Autodesk Inventor part; units mm, degrees
ref_plane "YZ Plane" through (0, 0, 0) normal (1, 0, 0) x (0, 1, 0)
ref_plane "XZ Plane" through (0, 0, 0) normal (0, 1, 0) x (-1, 0, 0)
ref_plane "XY Plane" through (0, 0, 0) normal (0, 0, 1) x (1, 0, 0)
sketch "Sketch1" plane through (0, 0, 0) normal (0, 1, 0) x (-1, 0, 0)
  line L0 (-3.6662, 6.35) -> (3.6662, 6.35)
  line L1 (3.6662, 6.35) -> (7.3323, 0)
  line L2 (7.3323, 0) -> (3.6662, -6.35)
  line L3 (3.6662, -6.35) -> (-3.6662, -6.35)
  line L4 (-3.6662, -6.35) -> (-7.3323, 0)
  line L5 (-7.3323, 0) -> (-3.6662, 6.35)
  point P0 (0, 0)
  point P1 (0, 0)
  dimension "d0" = 12.7
extrude "Extrusion1" add sketch "Sketch1" along normal blind 171.45
sketch "Sketch2" plane through (0, 171.45, 0) normal (0, 1, 0) x (1, 0, 0)
  circle A0 centre (0, 0) radius 2.54
  dimension "d3" = 5.08
extrude "Extrusion2" cut sketch "Sketch2" against normal blind 25.4
thread "Thread1"
sketch "Sketch3" plane through (0, 0, 0) normal (0, -1, 0) x (1, 0, 0)
  circle A0 centre (0, 0) radius 2.54
  dimension "d8" = 5.08
extrude "Extrusion3" cut sketch "Sketch3" against normal blind 25.4
thread "Thread2"
properties part number "OUTK_013_Shaft1" material "Aluminum 6061"
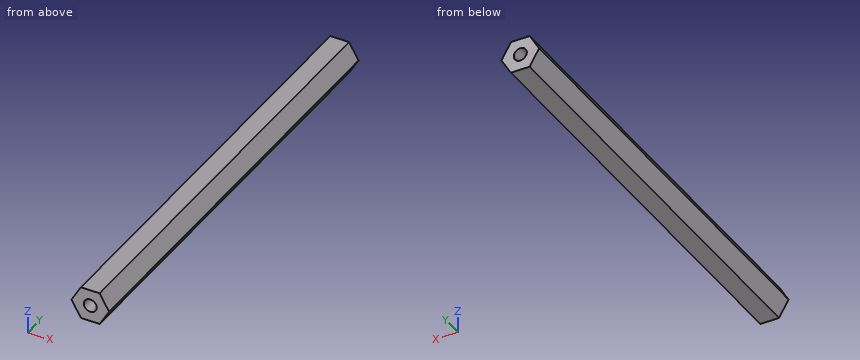
Source: CAD feature listing. Evaluate the final solid. Frame: model axes, mm. Give positions to 0.01 mm unless a question says otherwise; leave off trailing zeros. Loops run counter-clockwise (first coordinate to the right, second up) from the corner with the lowest first, then second, coordinate; pieces in that order, holes last. Notation, with made-up numbers: (42, 50) -> (76, 50) arc R20 ccw to (76, 58) -> close; hole circle Ø1 at (22, -23.75). An arc over 180 degrees is marked (long way). Use a Markdown table: item, result. Add a question column.
1) First-contact query: pin 1 (2.5 mm diameter, centred on x = 1, z = 0, fed in from +Y); pin 2 (4 mm diameter, centred on x = 0, z = 0, fed in from -Y); pin 3 (2 mm diameter, centred on x = 5, y = 51, fed in from +Z). Flat tips, straight axial feed; report the tip coordinate or a pass-through.
2) Section query A-A, the plane y = 150. Return the cut outline in (x, z), then the cut area to 3 significant figures.
3) Section query B-B, the plane y = 58. Return the cut outline in (x, z).
4) Section query C-C, the plane x = 0. Return the cut outline in (y, z).
5) Line query: line 1 along X through (y, z) = (152, 0); line 2 along Z through (x, y) = (0, 17.5); line 3 along Y through (x, z) = (-1.5, -2). Output: solid intervals per line, ascending. Write a range as [from, to].
Numbers:
| question | item | result |
|---|---|---|
| 1 | pin 1 | stops at y = 146.05 |
| 1 | pin 2 | stops at y = 25.4 |
| 1 | pin 3 | stops at z = 5.77 |
| 2 | outline | (-7.33, 0) -> (-3.67, -6.35) -> (3.67, -6.35) -> (7.33, 0) -> (3.67, 6.35) -> (-3.67, 6.35) -> close; hole circle Ø5.08 at (0, 0) |
| 2 | area | 119 mm2 |
| 3 | outline | (-7.33, 0) -> (-3.67, -6.35) -> (3.67, -6.35) -> (7.33, 0) -> (3.67, 6.35) -> (-3.67, 6.35) -> close |
| 4 | outline | (0, -6.35) -> (171.45, -6.35) -> (171.45, -2.54) -> (146.05, -2.54) -> (146.05, 2.54) -> (171.45, 2.54) -> (171.45, 6.35) -> (0, 6.35) -> (0, 2.54) -> (25.4, 2.54) -> (25.4, -2.54) -> (0, -2.54) -> close |
| 5 | line 1 | x = [-7.33, -2.54], [2.54, 7.33] |
| 5 | line 2 | z = [-6.35, -2.54], [2.54, 6.35] |
| 5 | line 3 | y = [25.4, 146.05] |
